Can you work these out from the drawing? Everything is in mm from the part's minimum corner. Give positions to 0.01 mm unless a question says otherwise; leave off trailing zeros. Order: outer loops, then holes, each group sorted by start corner. A loop starts at its lowest first (then second) coordinate and runs counter-clockwise, first axis right, second up. Notation, with made-up numbers: (49, -40) - (87, -40) arc R24 cw to (87, -12) - close; hole circle Ø7 at (-6.5, -12.5). An arc over 180 degrees is marked (long way). Answer as a JSON object with one key per item and string values.
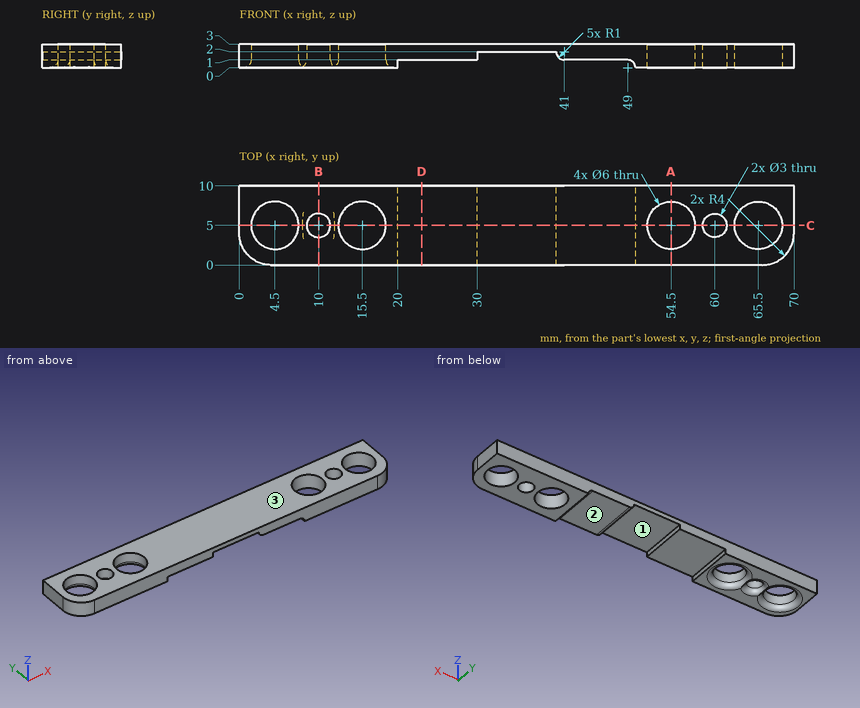
Q1. We'd pull the mould along X, two halves only. Please class the marked faces 1, 2 and 3: released by +X, released by -X, zero draft, split by the parting line, or undercut.
Recorded:
{"face 1": "undercut", "face 2": "undercut", "face 3": "zero draft"}
Q2. If we section it at D-D, the plane x = 23: Please give me the cut outline in (y, z).
Recorded:
{"outline": "(0, 1) - (10, 1) - (10, 3) - (0, 3) - close"}
Q3. If we section it at A-A, the plane x = 54.5: Please give me the cut outline in (y, z).
Recorded:
{"outline": "(0, 0) - (2, 0) - (2, 3) - (0, 3) - close; (8, 0) - (10, 0) - (10, 3) - (8, 3) - close"}
Q4. I'm going to push flat-ended pins straight in: pin 1 Ø3 at (x, y) = (26, 6.5) entering from -Z; pin 2 Ø2.5 at (x, y) = (60, 5) entering from +Z. Where does each tip first touch, or does it pass through?
Recorded:
{"pin 1": "stops at z = 1", "pin 2": "passes through"}
Q5. If we section it at C-C, the plane y = 5: Count the separate pieces of the cut face and the enclosed holes in it, then the cut area to 3 significant figures.
Recorded:
{"separate pieces": "7", "enclosed holes": "0", "area": "78.8 mm^2"}
Q6. I need wall thicknesses on L1, parallel to Y at x = 54.5, z = 1.3; L2, parallel to X at y = 3.25, z = 2.8; L3, parallel to Y at x = 60, z = 2. Which ranges of each line are inside material? Lowest first, please.
Recorded:
{"L1": "y = 0 to 2, 8 to 10", "L2": "x = 0.07 to 2.06, 6.94 to 13.06, 17.94 to 52.06, 56.94 to 63.06, 67.94 to 69.93", "L3": "y = 0 to 3.5, 6.5 to 10"}
Q7. If we section it at B-B, the plane x = 10: Please give me the cut outline in (y, z).
Recorded:
{"outline": "(0, 0) - (2.5, 0) arc R1 ccw to (3.5, 1) - (3.5, 3) - (0, 3) - close; (6.5, 1) arc R1 ccw to (7.5, 0) - (10, 0) - (10, 3) - (6.5, 3) - close"}
